Model file for the job. Use its own axes, mm. Face numbers are marked on the shaded views. A direction names the side the tool comes from. Coordinates: 2 decimals unless noted, no trailing zeros. Order: outer loops, then holes, each group sorted by start corner. A loop starts at its lowest first (then second) coordinate and runs counter-clockwise, first axis right, second up. Notation, with made-up numbers: (39.25, 11.5) -> (70.25, 11.5) arc R17 ccw to (70.25, 35.5) -> close; hole circle Ø2 at (35, 29). An arc over 180 degrees is marked (long way). Return JSON: item names as keys, results as strings. Group by question number.
1) Flat gauge pins, fed straight in: pin 1 (1.5 mm diameter, centred on y = -41, z = 10, fed in from -X); pin 2 (1 mm diameter, centred on y = -32, z = 14.5, fed in from -X); pin 3 (1 mm diameter, centred on x = -53, y = -21.5, fed in from -Z); pin 4 (3 mm diameter, centred on x = 8, z = 16.5, fed in from +Y). Where does each tip first touch, or does it go through?
2) Cut at C-C (y = -4). Write the cut outline in (x, z).
3) Pull direction X, two halves, no side cores. Call the marked faces 1, 2 and 3: +X half, -X half, draft (parallel to the pull), parting line (faces both ways), or undercut.
4) Cut at B-B (y = -23.5). Write the cut outline in (x, z), and give its area (3 significant figures).
5) Probe line 1 (X direction, y = 2.5, z = 16.5); line 2 (X direction, y = 27, z = 5.5); line 3 (X direction, y = 2, z = 8.75). List the from-to ranges inside material, lowest first.
6) Cut at D-D (x = 38.5). Write the cut outline in (y, z), and give its area (3 significant figures).
7) Which spindle directions (+Z, -Z, +X, -X, +Y, -Y) get a long thin tool onto all of the face, cutting with end or side? Do the marked faces 4, 5 and 6. Say none if no direction does.
8) Cut at A-A (z = 4.5). Write the cut outline in (x, y).
from build123d import *

# Parameters (mm, degrees)
AUFSATZ_LINEAR_AUSTRAGEN1_DEPTH = 20


with BuildPart() as part:
    # Skizze1 → Aufsatz-Linear austragen1 (new body)
    with BuildSketch(Plane.XY):
        with BuildLine():
            Line((-49.984452808, 20.068980322), (-69.984452808, 20.068980322))
            Line((-69.984452808, 20.068980322), (-69.984452808, 40.068980322))
            Line((-69.984452808, 40.068980322), (-82.468350795, 40.068980322))
            Line((-82.468350795, 40.068980322), (-82.468350795, -2.937308237))
            Line((-82.468350795, -2.937308237), (-82.468350795, -14.163354272))
            Line((-82.468350795, -14.163354272), (0, -61.776478803))
            Line((0, -61.776478803), (82.468350795, -14.163354272))
            Line((82.468350795, -14.163354272), (82.468350795, -2.937308237))
            Line((82.468350795, -2.937308237), (82.468350795, 40.068980322))
            Line((82.468350795, 40.068980322), (69.984452808, 40.068980322))
            Line((69.984452808, 40.068980322), (69.984452808, 20.068980322))
            Line((69.984452808, 20.068980322), (49.984452808, 20.068980322))
            Line((49.984452808, 20.068980322), (47.5, 0))
            ThreePointArc((47.5, 0), (0, -47.5), (-47.5, 0))
            Line((-47.5, 0), (-47.5, 10.568980322))
            Line((-47.5, 10.568980322), (-49.984452808, 20.068980322))
        make_face()
        Polygon((-59.984452808, 13.068980322), (-51, 7.881804075), (-51, -7.286243364), (-59.984452808, -12.47341961), (-68.968905615, -7.286243364), (-68.968905615, 7.881804075), align=None, mode=Mode.SUBTRACT)
    extrude(amount=AUFSATZ_LINEAR_AUSTRAGEN1_DEPTH)


solid = part.part
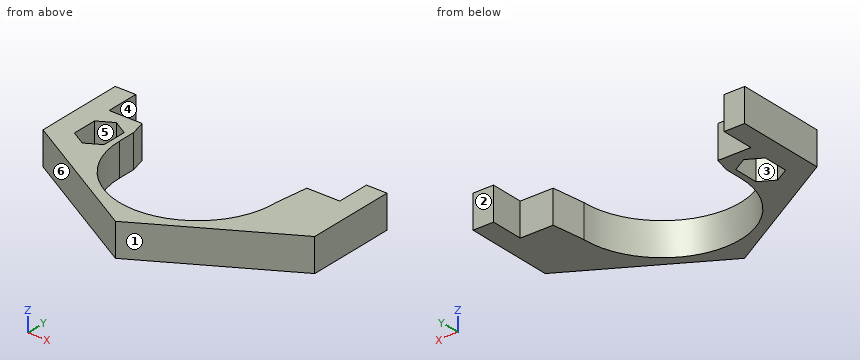
Answers below:
{
 "1": {"pin 1": "stops at x = -37.28", "pin 2": "stops at x = -52.44", "pin 3": "stops at z = 0", "pin 4": "stops at y = -46.54"},
 "2": {"outline": "(-82.47, 0) -> (-68.97, 0) -> (-68.97, 20) -> (-82.47, 20) -> close; (-51, 0) -> (-47.33, 0) -> (-47.33, 20) -> (-51, 20) -> close; (47.33, 0) -> (82.47, 0) -> (82.47, 20) -> (47.33, 20) -> close"},
 "3": {"face 1": "+X half", "face 2": "draft", "face 3": "undercut"},
 "4": {"outline": "(-66.3, 0) -> (-41.28, 0) -> (-41.28, 20) -> (-66.3, 20) -> close; (41.28, 0) -> (66.3, 0) -> (66.3, 20) -> (41.28, 20) -> close", "area": "1,000 mm^2"},
 "5": {"line 1": "x = -82.47 to -68.97, -51 to -47.5, 47.81 to 82.47", "line 2": "x = -82.47 to -69.98, 69.98 to 82.47", "line 3": "x = -82.47 to -68.97, -51 to -47.5, 47.75 to 82.47"},
 "6": {"outline": "(-39.55, 0) -> (-27.82, 0) -> (-27.82, 20) -> (-39.55, 20) -> close", "area": "235 mm^2"},
 "7": {"face 4": "+Z, -Z, +Y", "face 5": "+Z, -Z", "face 6": "+Z, -Z, -X, -Y"},
 "8": {"outline": "(-82.47, -14.16) -> (0, -61.78) -> (82.47, -14.16) -> (82.47, 40.07) -> (69.98, 40.07) -> (69.98, 20.07) -> (49.98, 20.07) -> (47.5, 0) arc R47.5 cw to (-47.5, 0) -> (-47.5, 10.57) -> (-49.98, 20.07) -> (-69.98, 20.07) -> (-69.98, 40.07) -> (-82.47, 40.07) -> close; hole (-68.97, -7.29) -> (-59.98, -12.47) -> (-51, -7.29) -> (-51, 7.88) -> (-59.98, 13.07) -> (-68.97, 7.88) -> close"}
}
